```python
from build123d import *

# Parameters (mm, degrees)
SKETCH1_W           = 25
SKETCH1_H           = 15
BOSS_EXTRUDE1_DEPTH = 20
SKETCH2_W           = 25
SKETCH2_H           = 14.55
CUT_EXTRUDE1_DEPTH  = 13
SKETCH4_R           = 2.55
BOSS_EXTRUDE2_DEPTH = 4.5
CHAMFER1_SIZE       = 1
SKETCH5_R           = 1.25
BOSS_EXTRUDE3_DEPTH = 2.5
CHAMFER2_SIZE       = 1


with BuildPart() as part:
    # Sketch1 → Boss-Extrude1 (new body)
    with BuildSketch(Plane.XY):
        with Locations((12.5, 7.5)):
            Rectangle(SKETCH1_W, SKETCH1_H)
    extrude(amount=BOSS_EXTRUDE1_DEPTH)

    # Sketch2 → Cut-Extrude1 (cut)
    with BuildSketch(Plane.XZ):
        with Locations((12.5, 10)):
            Rectangle(SKETCH2_W, SKETCH2_H)
    extrude(amount=-CUT_EXTRUDE1_DEPTH, mode=Mode.SUBTRACT)

    # Sketch4 → Boss-Extrude2 (add)
    with BuildSketch(Plane(origin=(0, 15, 0), x_dir=(1, 0, 0), z_dir=(0, 1, 0))):
        with Locations(Location((12.5, -10, 0), (0, 0, 270))):
            Circle(SKETCH4_R)
    extrude(amount=BOSS_EXTRUDE2_DEPTH)

    # Chamfer1
    chamfer1_edges = [part.edges().sort_by_distance(p)[0] for p in [
        (12.5, 19.5, 7.45),
    ]]
    chamfer(chamfer1_edges, length=CHAMFER1_SIZE)

    # Sketch5 → Boss-Extrude3 (add)
    with BuildSketch(Plane(origin=(0, 13, 0), x_dir=(-1, 0, 0), z_dir=(0, -1, 0))):
        with Locations(Location((-12.5, -10, 0), (0, 0, 180))):
            Circle(SKETCH5_R)
    extrude(amount=BOSS_EXTRUDE3_DEPTH)

    # Chamfer2
    chamfer2_edges = [part.edges().sort_by_distance(p)[0] for p in [
        (11.25, 10.5, 10),
    ]]
    chamfer(chamfer2_edges, length=CHAMFER2_SIZE)


solid = part.part
```
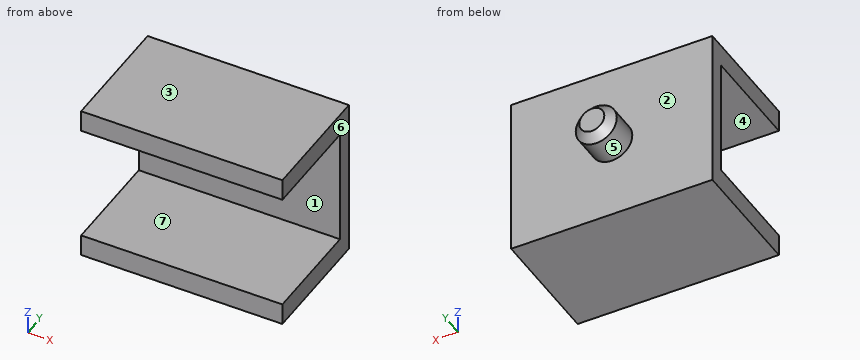
Model file for the job. Use its own axes, mm. Face numbers are marked on the shaded views. A direction names the side the tool comes from. Give positions to 0.01 mm unless a question says otherwise; leave off trailing zeros. Loops run counter-clockwise (first coordinate to the right, second up) from the corner with the lowest first, then second, coordinate; pieces in that order, holes last. Notation, with made-up numbers: (-14.75, 33.5) -> (-7.75, 33.5) arc R14 cw to (-7.75, 54.5) -> close; hole circle Ø11 at (83, 64). An arc over 180 degrees is marked (long way). Use CSV: the item, a comma, the result in double quotes. Start each with the question number.
1) Slice it at D-D on y = 17.25. Give the cut face in (x, z).
2) Tool access for the marked faces 5, 6 and 7: list every direction of +Z, -Z, +X, -X, +Y, -Y with a clear straight run to the whole face (end or side of a thin tool).
3) Slice it at B-B on x = 7. Give the cut face in (y, z) (3 decimals), plus the area to 3 significant figures.
4) Mould opens along Z. For the marked faces 1, 2, 3 and 4 say: released by +Z, released by -Z, zero draft, split by the parting line, or undercut.
5) Slice it at A-A on y = 6. Give the cut face in (x, z) (3 decimals), plus the area to 3 significant figures.
6) Wall check: line 1 (Z direction, x = 19.75, y = 4.75) (3 decimals); line 2 (Y direction, x = 16, z = 5.5); line 3 (Y direction, x = 6.75, z = 1). Give the ranges that are in metal, low to high.
7) Slice it at C-C on z = 3.75. Give the cut face in (x, y).
8) Flat gauge pin, fed straight in: pin 1 Ø2 at (x, z) = (8.5, 12) entering from +Y. Where does the tip first touch, or does it go through?
Computed values:
1,outline,"circle Ø5.1 at (12.5, 10)"
2,face 5,"+Y"
2,face 6,"+Z, -Z, +X, +Y, -Y"
2,face 7,"+X, -X, -Y"
3,outline,"(0, 0) -> (15, 0) -> (15, 20) -> (0, 20) -> (0, 17.275) -> (13, 17.275) -> (13, 2.725) -> (0, 2.725) -> close"
3,area,"111 mm^2"
4,face 1,"undercut"
4,face 2,"zero draft"
4,face 3,"released by +Z"
4,face 4,"undercut"
5,outline,"(0, 0) -> (25, 0) -> (25, 2.725) -> (0, 2.725) -> close; (0, 17.275) -> (25, 17.275) -> (25, 20) -> (0, 20) -> close"
5,area,"136 mm^2"
6,line 1,"z = 0 to 2.725, 17.275 to 20"
6,line 2,"y = 13 to 15"
6,line 3,"y = 0 to 15"
7,outline,"(0, 13) -> (25, 13) -> (25, 15) -> (0, 15) -> close"
8,pin 1,"stops at y = 15"
